For this review, take the finished solid that the model builds, in its own axes (mm). Face numbers are marked on the shaded views. A direction names the side the tool comes from. Coordinates: 2 decimals unless noted, no trailing zeros. Loops run counter-clockwise (first coordinate to the right, second up) from the corner with the lowest first, then second, coordinate; pieces in that order, holes last. Notation, with made-up numbers: M -33,0.5 L -13,0.5 A14 cw -13,9.5 Z; hole C 12.25,-14 d1. An arc over 180 degrees is marked long. Put each result on its own line as item: value.
```python
from build123d import *

# Parameters (mm, degrees)
SKETCH2_W           = 75
SKETCH2_H           = 80
SKETCH2_W_2         = 17.5
SKETCH2_H_2         = 76
SKETCH2_W_3         = 16.5
SKETCH2_W_4         = 15.5
BOSS_EXTRUDE1_DEPTH = 18
SKETCH3_W           = 75
SKETCH3_H           = 80
BOSS_EXTRUDE3_DEPTH = 2
SKETCH4_R           = 1.5
CUT_EXTRUDE1_DEPTH  = 3


with BuildPart() as part:
    # Sketch2 → Boss-Extrude1 (new body)
    with BuildSketch(Plane(origin=(0, 0, 0), x_dir=(1, 0, 0), z_dir=(0, 1, 0))):
        Rectangle(SKETCH2_W, SKETCH2_H)
        with Locations((-26.75, 0)):
            Rectangle(SKETCH2_W_2, SKETCH2_H_2, mode=Mode.SUBTRACT)
        with Locations((27.25, 0)):
            Rectangle(SKETCH2_W_3, SKETCH2_H_2, mode=Mode.SUBTRACT)
        with Locations((-8.25, 0)):
            Rectangle(SKETCH2_W_4, SKETCH2_H_2, mode=Mode.SUBTRACT)
        with Locations((9.25, 0)):
            Rectangle(SKETCH2_W_4, SKETCH2_H_2, mode=Mode.SUBTRACT)
    extrude(amount=BOSS_EXTRUDE1_DEPTH)

    # Sketch3 → Boss-Extrude3 (add)
    with BuildSketch(Plane.XZ):
        Rectangle(SKETCH3_W, SKETCH3_H)
    extrude(amount=BOSS_EXTRUDE3_DEPTH)

    # Sketch4 → Cut-Extrude1 (cut, through all)
    with BuildSketch(Plane(origin=(0, 0, 0), x_dir=(1, 0, 0), z_dir=(0, 1, 0))):
        with Locations((-26.75, -0.5)):
            Circle(SKETCH4_R)
    cut_extrude1 = extrude(amount=-CUT_EXTRUDE1_DEPTH, mode=Mode.SUBTRACT)

    # Mirror1: Cut-Extrude1 across plane
    add(cut_extrude1.mirror(Plane(origin=(0, 0, 0), x_dir=(0, 0, 1), z_dir=(1, 0, 0))), mode=Mode.SUBTRACT)


solid = part.part
```
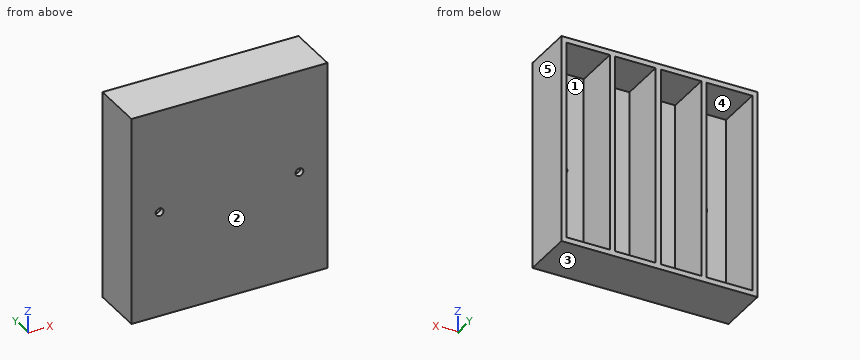
(1) Add section D-D (x = -10). Write out the cut boundary in (y, z), plus the area to 3 significant figures.
Determined:
outline: M -2,-40 L 18,-40 L 18,-38 L 0,-38 L 0,38 L 18,38 L 18,40 L -2,40 Z
area: 232 mm^2
(2) For pin 1 (2.5 mm diameter, centred on x = 26.75, z = 0.5, fed in from -Y); pin 2 (5 mm diameter, centred on x = -26.5, z = -0.5, fed in from +Y), all flat-tipped, find the tip position at first contact; note any pin that passes through.
Determined:
pin 1: passes through
pin 2: stops at y = 0
(3) Add section B-B (z = 0.5). Write out the cut boundary in (x, y).
Determined:
outline: M -37.5,-2 L -28.25,-2 L -28.25,0 L -35.5,0 L -35.5,18 L -37.5,18 Z; M -25.25,-2 L 25.25,-2 L 25.25,0 L 19,0 L 19,18 L 17,18 L 17,0 L 1.5,0 L 1.5,18 L -0.5,18 L -0.5,0 L -16,0 L -16,18 L -18,18 L -18,0 L -25.25,0 Z; M 28.25,-2 L 37.5,-2 L 37.5,18 L 35.5,18 L 35.5,0 L 28.25,0 Z
(4) Wall thickness on line 1 along X through (y, z) = (-0.9, 0.5); line 2 along X through (y, z) = (8.25, -25); line 3 along Z through (x, y) = (-8, 5.5): over which ranges is each line inside the solid? List them lowest first. Write a range as [from, to].
Determined:
line 1: x = [-37.5, -28.25], [-25.25, 25.25], [28.25, 37.5]
line 2: x = [-37.5, -35.5], [-18, -16], [-0.5, 1.5], [17, 19], [35.5, 37.5]
line 3: z = [-40, -38], [38, 40]
(5) Add section A-A (x = 26.75). Write out the cut boundary in (y, z).
Determined:
outline: M -2,-40 L 18,-40 L 18,-38 L 0,-38 L 0,-1 L -2,-1 Z; M -2,2 L 0,2 L 0,38 L 18,38 L 18,40 L -2,40 Z
(6) Draft analysis for pull direction Z (two halves, no side actions). For the marked faces 3, 4 and 5, state which applies: +Z half, -Z half, draft (parallel to the pull), parting line (faces both ways), or undercut.
Determined:
face 3: -Z half
face 4: undercut
face 5: draft
(7) Add section C-C (y = 13). Write out the cut boundary in (x, z).
Determined:
outline: M -37.5,-40 L 37.5,-40 L 37.5,40 L -37.5,40 Z; hole M -35.5,-38 L -18,-38 L -18,38 L -35.5,38 Z; hole M -16,-38 L -0.5,-38 L -0.5,38 L -16,38 Z; hole M 1.5,-38 L 17,-38 L 17,38 L 1.5,38 Z; hole M 19,-38 L 35.5,-38 L 35.5,38 L 19,38 Z
(8) Tool access review of the marked faces 1 and 2: name each direction out of +Z, -Z, +X, -X, +Y, -Y from which nothing blocks a thin tool from reaching the whole face with its end or side.
Determined:
face 1: +Y
face 2: +Z, -Z, +X, -X, -Y
